Can you work these out from the model? Positions are in its coordinate system, mm. A direction names the side the tool comes from. Give positions to 0.01 mm unless a question says otherwise; leave off trailing zeros. Loops run counter-clockwise (first coordinate to the right, second up) from the corner with the lowest first, then second, coordinate; pieces in that order, holes last. Notation, with made-up numbers: (21.5, 33) - (28.5, 33) arc R18 cw to (28.5, 55) - close; hole circle Ø6 at (-22.75, 41). An arc over 180 degrees is marked (long way). Answer as a JSON object with one key per item and string values. Group by question number.
Item 1: Please list where these lines run through material, in increasing order: L1, parallel to X at y = -54.5, z = 19.5; L2, parallel to Y at x = -15.5, z = 23.5; L3, parallel to Z at x = -2.5, y = -20.
Item 2: Will these pins go through, and if not, where does the flat tip stop? pin 1 (7.5 mm diameter, centred on x = -28.5, y = -70.5, fed in from -Z); pin 2 (10 mm diameter, centred on x = -5.5, z = 23, fed in from -Y); pin 3 (5 mm diameter, centred on x = -20.5, y = -11, fed in from -Z).
Item 3: Thinking about a two-plate mould opening in Z: for faces 4 (the flat face through (-28, -90, 31)), 5 (the cylindrical face through (-6.891, -14.79, -33.087)), 6 (the cylindrical face through (-28.4, -79.33, 40.26)), which applies, pulls with the +Z half, pulls with the -Z half, needs draft (parallel to the pull), parting line crosses it, or undercut?
Item 4: Suppose I cut it at C-C on y = -46.5. Write out the boundary of the cut face in (x, z).
Item 5: Which directions (+Z, -Z, +X, -X, +Y, -Y) give clear straight access to the entire face, cutting with the end or side of a thin tool? Please do faces 1 (the flat face through (11.656, -60, 31)), 2 (the cylindrical face through (-1.504, -14.79, 3.899)), 3 (the flat face through (16, -57, 12.646)).
Item 6: Suppose I cut it at A-A on z = -1. Write out the boundary of the cut face in (x, y).
Item 7: Suppose I cut it at D-D on z = 37. Write out the boundary of the cut face in (x, y).
Item 8: Suppose I cut it at B-B on y = -20.5. Write out the boundary of the cut face in (x, z), and give its area (3 significant figures).
from build123d import *

# Parameters (mm, degrees)
F1_DEPTH = 30
F2_W     = 6.907336
F2_H     = 37
F2_W_2   = 8.058561
F3_DEPTH = 60
F4_R     = 5
F5_R     = 8.388912
F6_DEPTH = 30
F7_R     = 7.936713
F8_DEPTH = 30


with BuildPart() as f1:
    # F0 (on Front) → F1 (new body)
    with BuildSketch(Plane.XZ):
        with BuildLine():
            Line((19.714694, 49.646493), (-31.802535, 49.646493))
            Line((-31.802535, 49.646493), (-31.802535, -7.339047))
            ThreePointArc((-31.802535, -7.339047), (-6.328528, -33.099269), (19.714694, -7.914659))
            Line((19.714694, -7.914659), (19.714694, 49.646493))
        make_face()
        with BuildLine():
            ThreePointArc((-12.231744, 0.324407), (-10.767278, 3.85994), (-7.231744, 5.324407))
            Line((-7.231744, 5.324407), (-5, 5.324407))
            ThreePointArc((-5, 5.324407), (-1.464466, 3.85994), (0, 0.324407))
            Line((0, 0.324407), (0, -20.758615))
            ThreePointArc((0, -20.758615), (-1.464466, -24.294149), (-5, -25.758615))
            Line((-5, -25.758615), (-7.231744, -25.758615))
            ThreePointArc((-7.231744, -25.758615), (-10.767278, -24.294149), (-12.231744, -20.758615))
            Line((-12.231744, -20.758615), (-12.231744, 0.324407))
        make_face(mode=Mode.SUBTRACT)
    extrude(amount=F1_DEPTH)

    # F2 (on face) → F3 (join)
    with BuildSketch(Plane.XZ.offset(30)):
        with Locations((-28.348867, 31.146493)):
            Rectangle(F2_W, F2_H)
        with Locations((15.685413, 31.146493)):
            Rectangle(F2_W_2, F2_H)
    extrude(amount=F3_DEPTH)

    # F4
    f4_edges = [f1.edges().sort_by_distance(p)[0] for p in [
        (15.685413, -90, 49.646493),
        (15.685413, -90, 12.646493),
        (-28.348867, -90, 49.646493),
        (-28.348867, -90, 12.646493),
    ]]
    fillet(f4_edges, radius=F4_R)

    # F5 (on face) → F6 (cut)
    with BuildSketch(Plane.YZ.offset(19.714694)):
        with Locations((-73.927611, 33.851173)):
            Circle(F5_R)
    extrude(amount=-F6_DEPTH, mode=Mode.SUBTRACT)

    # F7 (on face) → F8 (cut)
    with BuildSketch(Plane(origin=(-31.802535, 0, 0), x_dir=(0, -1, 0), z_dir=(-1, 0, 0))):
        with Locations((75.060703, 33.567894)):
            Circle(F7_R)
    extrude(amount=-F8_DEPTH, mode=Mode.SUBTRACT)


solid = f1.part
Worked out:
{
 "1": {"L1": "x = -31.8 to -24.9, 11.66 to 19.71", "L2": "y = -30 to 0", "L3": "z = -32.86 to -25.09, 4.65 to 49.65"},
 "2": {"pin 1": "stops at z = 12.65", "pin 2": "stops at y = -30", "pin 3": "stops at z = -30.16"},
 "3": {"face 4": "needs draft", "face 5": "pulls with the -Z half", "face 6": "undercut"},
 "4": {"outline": "(-31.8, 12.65) - (-24.9, 12.65) - (-24.9, 49.65) - (-31.8, 49.65) - close; (11.66, 12.65) - (19.71, 12.65) - (19.71, 49.65) - (11.66, 49.65) - close"},
 "5": {"face 1": "+Z, -Z, -Y", "face 2": "+Y, -Y", "face 3": "-Z, +X, -X, -Y"},
 "6": {"outline": "(-31.8, -30) - (-12.23, -30) - (-12.23, 0) - (-31.8, 0) - close; (0, -30) - (19.71, -30) - (19.71, 0) - (0, 0) - close"},
 "7": {"outline": "(-31.8, -90) - (-24.9, -90) - (-24.9, -82.22) - (-31.8, -82.22) - close; (-31.8, -67.9) - (-24.9, -67.9) - (-24.9, -30) - (11.66, -30) - (11.66, -66.15) - (19.71, -66.15) - (19.71, 0) - (-31.8, 0) - close; (11.66, -90) - (19.71, -90) - (19.71, -81.7) - (11.66, -81.7) - close"},
 "8": {"outline": "(-31.8, -7.34) arc R25.76 ccw to (19.71, -7.91) - (19.71, 49.65) - (-31.8, 49.65) - close; hole (-12.23, -20.76) arc R5 ccw to (-7.23, -25.76) - (-5, -25.76) arc R5 ccw to (0, -20.76) - (0, 0.32) arc R5 ccw to (-5, 5.32) - (-7.23, 5.32) arc R5 ccw to (-12.23, 0.32) - close", "area": "3,620 mm2"}
}
